```python
from build123d import *

# Parameters (mm, degrees)
F0_W      = 20
F0_H      = 660
F0_H_2    = 20
F1_DEPTH  = 20
F2_DEPTH  = 680
F3_W      = 20
F3_H      = 20
F4_DEPTH  = 660
F5_W      = 20
F5_H      = 20
F6_DEPTH  = 680
F7_W      = 20
F7_H      = 20
F8_DEPTH  = 660
F9_W      = 20
F9_H      = 20
F10_DEPTH = 660


with BuildPart() as f1:
    # F0 (on Top) → F1 (new body)
    with BuildSketch(Plane.XY):
        Polygon((350.936165, 480.516352), (-329.063835, 480.516352), (-329.063835, 460.516352), (330.936165, 460.516352), (330.936165, -199.483648), (-329.063835, -199.483648), (-329.063835, -219.483648), (350.936165, -219.483648), align=None)
        with Locations((-339.063835, 130.516352)):
            Rectangle(F0_W, F0_H)
        with Locations((-339.063835, 470.516352)):
            Rectangle(F0_W, F0_H_2)
        with Locations((-339.063835, -209.483648)):
            Rectangle(F0_W, F0_H_2)
    extrude(amount=F1_DEPTH)

    # F0 (on Top) → F2 (join)
    with BuildSketch(Plane.XY):
        with Locations((-339.063835, 470.516352)):
            Rectangle(F0_W, F0_H_2)
        with Locations((-339.063835, -209.483648)):
            Rectangle(F0_W, F0_H_2)
    extrude(amount=F2_DEPTH)

    # F3 (on face) → F4 (join)
    with BuildSketch(Plane(origin=(0, -199.483648, 0), x_dir=(-1, 0, 0), z_dir=(0, 1, 0))):
        with Locations((339.063835, 670)):
            Rectangle(F3_W, F3_H)
    extrude(amount=F4_DEPTH)

    # F5 (on face) → F6 (join)
    with BuildSketch(Plane.YZ.offset(-329.063835)):
        with Locations((-209.483648, 670)):
            Rectangle(F5_W, F5_H)
        with Locations((470.516352, 670)):
            Rectangle(F5_W, F5_H)
    extrude(amount=F6_DEPTH)

    # F7 (on face) → F8 (join)
    with BuildSketch(Plane.XY.offset(20)):
        with Locations((340.936165, 470.516352)):
            Rectangle(F7_W, F7_H)
        with Locations((340.936165, -209.483648)):
            Rectangle(F7_W, F7_H)
    extrude(amount=F8_DEPTH)

    # F9 (on face) → F10 (join)
    with BuildSketch(Plane.XZ.offset(-460.516352)):
        with Locations((340.936165, 670)):
            Rectangle(F9_W, F9_H)
    extrude(amount=F10_DEPTH)


solid = f1.part
```
Input: part model. Units: mm. Frame: model coordinates. A direction names the side the tool comes from. Give positions to 0.01 mm unless a question says otherwise; leave off trailing zeros. Order: outer loops, then holes, each group sorted by start corner. A loop starts at its lowest first (then second) coordinate and runs counter-clockwise, first axis right, second up.
1. Cut plane A-A (x = -14). Return loops of the section in (y, z), and give its area (3 significant figures).
Computed:
outline: (-219.48, 0) - (-199.48, 0) - (-199.48, 20) - (-219.48, 20) - close; (-219.48, 660) - (-199.48, 660) - (-199.48, 680) - (-219.48, 680) - close; (460.52, 0) - (480.52, 0) - (480.52, 20) - (460.52, 20) - close; (460.52, 660) - (480.52, 660) - (480.52, 680) - (460.52, 680) - close
area: 1,600 mm2
2. Set-up query: faces 1 (the face through (341, 135, 660)), 2 (the face through (330.936, -210, 336)), 3 (the face through (-4, 460.516, 10)). Return all of +Z, -Z, +X, -X, +Y, -Y with unobstructed straight access to the full face (end or side cutting, diameter ignored); none if empty.
Computed:
face 1: +X, -X
face 2: +Y, -Y
face 3: +Z, -Z
3. Cut plane B-B (z = 84.5). Return loops of the section in (x, y).
Computed:
outline: (-349.06, -219.48) - (-329.06, -219.48) - (-329.06, -199.48) - (-349.06, -199.48) - close; (-349.06, 460.52) - (-329.06, 460.52) - (-329.06, 480.52) - (-349.06, 480.52) - close; (330.94, -219.48) - (350.94, -219.48) - (350.94, -199.48) - (330.94, -199.48) - close; (330.94, 460.52) - (350.94, 460.52) - (350.94, 480.52) - (330.94, 480.52) - close
4. Draft query along Y for faces 4 (the face through (-27, -205, 680)), 5 (the face through (-339, 135, 20)), 6 (the face through (-1, -219.484, 11)). Return one class per face: released by +Y, released by -Y, zero draft, split by the parting line, or undercut.
Computed:
face 4: zero draft
face 5: undercut
face 6: released by -Y
